The listing builds one solid part. Answer for the finished solid, in the listing's coordinates (mm). Coordinates: 2 decimals unless noted, no trailing zeros. Order: outer loops, then holes, each group sorted by start corner. A loop starts at its lowest first (then second) coordinate and runs counter-clockwise, first axis right, second up. Notation, with made-up numbers: (53.5, -26.5) -> (104.5, -26.5) arc R7 cw to (104.5, -20.5) -> close; hole circle Ø1 at (-5, 5). An arc over 180 degrees is marked (long way). Write each question's results on one line, items separated by ' | '. Start each with the question number.
(1) Straight lines are drawn through the part: L1, parallel to Z at x = -18.5, y = 0; L2, parallel to Z at x = -7.5, y = 19. For each, find the intervals that lie inside material, in ascending order.
(2) The part is cut by section B-B, the plane y = 10. Give the vertices of the cut face in (x, z).
(3) The part is cut by section A-A, the plane z = 0. Give the vertices of the cut face in (x, y), then the cut area to 3 significant figures.
(4) Given pin 1 (4 mm diameter, centred on x = 7, y = 5, fed in from +Z), flat-ended and moving along its own axis, determine where the tip first touches the part or whether it passes through.
(5) Determine the mould class of faces 1 (the face through (23.59, -0.27, -23.49)), 2 (the face through (-8.88, -15.98, 0.39)), 3 (the face through (8, 25.4, 5)), 4 (the face through (-23.59, -23.49, 0.27)) for opening direction X: +X half, -X half, draft (parallel to the pull), parting line (faces both ways), or undercut.
```python
from build123d import *

# Parameters (mm, degrees)
F0_W     = 50.8
F0_H     = 50.8
F1_DEPTH = 25.4
F2_R     = 6.35
F3_R     = 8.89
F4_DEPTH = 50.8
F5_R     = 8.89
F6_DEPTH = 50.8
F7_R     = 8.89
F8_DEPTH = 50.8


with BuildPart() as f1:
    # F0 (on Front) → F1 (new body, symmetric)
    with BuildSketch(Plane.XZ):
        Rectangle(F0_W, F0_H)
    extrude(amount=F1_DEPTH, both=True)

    # F2
    f2_edges = [f1.edges().sort_by_distance(p)[0] for p in [
        (0, -25.4, 25.4),
        (25.4, 0, 25.4),
        (25.4, 0, -25.4),
        (0, -25.4, -25.4),
        (25.4, -25.4, 0),
        (0, 25.4, 25.4),
        (-25.4, 0, 25.4),
        (25.4, 25.4, 0),
        (-25.4, -25.4, 0),
        (-25.4, 0, -25.4),
        (-25.4, 25.4, 0),
        (0, 25.4, -25.4),
    ]]
    fillet(f2_edges, radius=F2_R)

    # F3 (on face) → F4 (cut, through all)
    with BuildSketch(Plane.XY.offset(25.4)):
        Circle(F3_R)
    extrude(amount=-F4_DEPTH, mode=Mode.SUBTRACT)

    # F5 (on face) → F6 (cut, through all)
    with BuildSketch(Plane.XZ.offset(25.4)):
        Circle(F5_R)
    extrude(amount=-F6_DEPTH, mode=Mode.SUBTRACT)

    # F7 (on face) → F8 (cut, through all)
    with BuildSketch(Plane.YZ.offset(25.4)):
        Circle(F7_R)
    extrude(amount=-F8_DEPTH, mode=Mode.SUBTRACT)


solid = f1.part
```
Established:
1) L1: z = -25.4 to -8.89, 8.89 to 25.4 | L2: z = -25.4 to -4.77, 4.77 to 25.4
2) outline: (-25.4, -19.05) arc R6.35 ccw to (-19.05, -25.4) -> (19.05, -25.4) arc R6.35 ccw to (25.4, -19.05) -> (25.4, 19.05) arc R6.35 ccw to (19.05, 25.4) -> (-19.05, 25.4) arc R6.35 ccw to (-25.4, 19.05) -> close; hole circle Ø17.78 at (0, 0)
3) outline: (-25.4, -19.05) arc R6.35 ccw to (-19.05, -25.4) -> (-8.89, -25.4) -> (-8.89, -8.89) -> (-25.4, -8.89) -> close; (-25.4, 8.89) -> (-8.89, 8.89) -> (-8.89, 25.4) -> (-19.05, 25.4) arc R6.35 ccw to (-25.4, 19.05) -> close; (8.89, -25.4) -> (19.05, -25.4) arc R6.35 ccw to (25.4, -19.05) -> (25.4, -8.89) -> (8.89, -8.89) -> close; (8.89, 8.89) -> (25.4, 8.89) -> (25.4, 19.05) arc R6.35 ccw to (19.05, 25.4) -> (8.89, 25.4) -> close | area: 1,060 mm^2
4) pin 1: stops at z = 25.4
5) face 1: +X half | face 2: undercut | face 3: draft | face 4: -X half
